from build123d import *

# Parameters (mm, degrees)
SKETCH1_W                = 154.8
SKETCH1_H                = 121.9997
SKETCH1_R                = 2.2
BOSS_EXTRUDE1_DEPTH      = 10
SKETCH2_W                = 184.8
SKETCH2_H                = 151.9997
SKETCH2_W_2              = 154.8
SKETCH2_H_2              = 121.9997
BOSS_EXTRUDE2_DEPTH      = 18
SKETCH2_2_W              = 184.8
SKETCH2_2_H              = 151.9997
SKETCH2_2_W_2            = 154.8
SKETCH2_2_H_2            = 121.9997
BOSS_EXTRUDE3_DEPTH      = 5
CUT_EXTRUDE1_DEPTH       = 229.604349915
CUT_EXTRUDE2_REACH       = 232.747
M5_CLEARANCE_HOLE1_D     = 5.5
M5_CLEARANCE_HOLE1_DEPTH = 23
M5_CLEARANCE_HOLE1_TIP   = 1.652366702
CUT_EXTRUDE3_DEPTH       = 6
CHAMFER1_SIZE            = 1
CHAMFER2_SIZE            = 3


with BuildPart() as part:
    # Sketch1 → Boss-Extrude1 (new body)
    with BuildSketch(Plane(origin=(0, 0, 0), x_dir=(1, 0, 0), z_dir=(0, 1, 0))):
        with Locations((77.4, 60.99985)):
            Rectangle(SKETCH1_W, SKETCH1_H)
        with Locations(Location((10, 53.3997, 0), (0, 0, 270))):
            Circle(SKETCH1_R, mode=Mode.SUBTRACT)
        with Locations(Location((10, 94.3997, 0), (0, 0, 270))):
            Circle(SKETCH1_R, mode=Mode.SUBTRACT)
        with Locations(Location((102, 94.3997, 0), (0, 0, 270))):
            Circle(SKETCH1_R, mode=Mode.SUBTRACT)
        with Locations(Location((102, 53.3997, 0), (0, 0, 270))):
            Circle(SKETCH1_R, mode=Mode.SUBTRACT)
        with BuildLine():
            Line((8, 49.3997), (8, 25.4))
            Line((8, 25.4), (104, 25.4))
            Line((104, 25.4), (104, 49.706462937))
            ThreePointArc((104, 49.706462937), (97.8, 53.3997), (104, 57.092937063))
            Line((104, 57.092937063), (104, 90.706462937))
            ThreePointArc((104, 90.706462937), (98.94961445, 91.512634363), (98.422291236, 96.5997))
            Line((98.422291236, 96.5997), (47, 96.5997))
            Line((47, 96.5997), (47, 49.3997))
            Line((47, 49.3997), (8, 49.3997))
        make_face(mode=Mode.SUBTRACT)
    extrude(amount=BOSS_EXTRUDE1_DEPTH)

    # Sketch2 → Boss-Extrude2 (add)
    with BuildSketch(Plane.XZ):
        with Locations((77.4, -60.99985)):
            Rectangle(SKETCH2_W, SKETCH2_H)
        with Locations((77.4, -60.99985)):
            Rectangle(SKETCH2_W_2, SKETCH2_H_2, mode=Mode.SUBTRACT)
    extrude(amount=-BOSS_EXTRUDE2_DEPTH)

    # Sketch2<2> → Boss-Extrude3 (add)
    # profile 1 of 2: a face of its own
    with BuildSketch(Plane.XZ):
        with Locations((77.4, -60.99985)):
            Rectangle(SKETCH2_2_W, SKETCH2_2_H)
        with Locations((77.4, -60.99985)):
            Rectangle(SKETCH2_2_W_2, SKETCH2_2_H_2, mode=Mode.SUBTRACT)
    # profile 2 of 2: a face of its own
    with BuildSketch(Plane.XZ):
        with Locations((77.4, -60.99985)):
            Rectangle(SKETCH2_2_W_2, SKETCH2_2_H_2)
    extrude(amount=BOSS_EXTRUDE3_DEPTH)

    # Sketch3 → Cut-Extrude1 (cut, through all)
    with BuildSketch(Plane.XY.offset(15)):
        with BuildLine():
            Line((52.4, 22), (102.4, 22))
            ThreePointArc((102.4, 22), (106.4, 18), (102.4, 14))
            Line((102.4, 14), (52.4, 14))
            ThreePointArc((52.4, 14), (48.4, 18), (52.4, 22))
        make_face()
    extrude(amount=-CUT_EXTRUDE1_DEPTH, mode=Mode.SUBTRACT)

    # Sketch4 → Cut-Extrude2 (cut, up to next)
    with BuildSketch(Plane(origin=(169.8, 0, 0), x_dir=(0, 0, -1), z_dir=(1, 0, 0)), mode=Mode.PRIVATE) as cut_extrude2_sk1:
        with BuildLine():
            Line((50.99985, 24), (70.99985, 24))
            ThreePointArc((70.99985, 24), (76.99985, 18), (70.99985, 12))
            Line((70.99985, 12), (50.99985, 12))
            ThreePointArc((50.99985, 12), (44.99985, 18), (50.99985, 24))
        make_face()
    cut_extrude2_tool1 = extrude(cut_extrude2_sk1.sketch, amount=-CUT_EXTRUDE2_REACH, mode=Mode.PRIVATE) & part.part
    add(cut_extrude2_tool1.solids().sort_by_distance((169.8, 18, -60.99985))[0], mode=Mode.SUBTRACT)

    # M5 Clearance Hole1
    with Locations(Plane(origin=(0, 18, 0), x_dir=(1, 0, 0), z_dir=(0, 1, 0))):
        with Locations((162.3, 129.4997), (162.3, -7.5), (-7.5, 129.4997), (-7.5, -7.5)):
            Hole(M5_CLEARANCE_HOLE1_D / 2, depth=M5_CLEARANCE_HOLE1_DEPTH)
            with Locations((0, 0, -(M5_CLEARANCE_HOLE1_DEPTH + M5_CLEARANCE_HOLE1_TIP / 2))):  # 118° drill point
                Cone(0, M5_CLEARANCE_HOLE1_D / 2, M5_CLEARANCE_HOLE1_TIP, mode=Mode.SUBTRACT)

    # Sketch7 → Cut-Extrude3 (cut)
    with BuildSketch(Plane.XZ.offset(5)):
        Polygon((-3.4, 9.867136104), (-7.5, 12.234272207), (-11.6, 9.867136104), (-11.6, 5.132863896), (-7.5, 2.765727793), (-3.4, 5.132863896), align=None)
        Polygon((158.2, 9.867136104), (158.2, 5.132863896), (162.3, 2.765727793), (166.4, 5.132863896), (166.4, 9.867136104), (162.3, 12.234272207), align=None)
        Polygon((158.2, -127.132563896), (158.2, -131.866836104), (162.3, -134.233972207), (166.4, -131.866836104), (166.4, -127.132563896), (162.3, -124.765427793), align=None)
        Polygon((-3.4, -127.132563896), (-7.5, -124.765427793), (-11.6, -127.132563896), (-11.6, -131.866836104), (-7.5, -134.233972207), (-3.4, -131.866836104), align=None)
    extrude(amount=-CUT_EXTRUDE3_DEPTH, mode=Mode.SUBTRACT)

    # Chamfer1
    chamfer1_edges = [part.edges().sort_by_distance(p)[0] for p in [
        (77.4, 14, 0),
        (77.4, 14, -121.9997),
        (49.571572875, 15.171572875, -121.9997),
        (49.571572875, 15.171572875, 0),
        (105.228427125, 15.171572875, 0),
        (105.228427125, 15.171572875, -121.9997),
        (154.8, 10, -60.99985),
        (154.8, 12, -60.99985),
        (154.8, 13.757359313, -46.757209313),
        (154.8, 13.757359313, -75.242490687),
        (77.4, 10, -121.9997),
        (27.5, 0, -49.3997),
        (47, 5, -49.3997),
        (8, 0, -37.39985),
        (8, 5, -49.3997),
        (56, 0, -25.4),
        (8, 5, -25.4),
        (104, 0, -37.553231469),
        (104, 5, -25.4),
        (97.8, 0, -53.3997),
        (104, 0, -73.8997),
        (98.94961445, 0, -91.512634363),
        (72.711145618, 0, -96.5997),
        (47, 0, -72.9997),
        (47, 5, -96.5997),
        (27.5, 10, -49.3997),
        (8, 10, -37.39985),
        (56, 10, -25.4),
        (104, 10, -37.553231469),
        (104, 10, -73.8997),
        (72.711145618, 10, -96.5997),
        (47, 10, -72.9997),
        (0, 10, -60.99985),
        (154.8, 14, 0),
        (0, 14, -121.9997),
        (0, 14, 0),
        (154.8, 14, -121.9997),
        (-15, 6.5, 15),
        (169.8, 6.5, 15),
        (169.8, 6.5, -136.9997),
        (-15, 6.5, -136.9997),
        (169.8, -5, -60.99985),
        (77.4, -5, 15),
        (77.4, 10, 0),
        (-15, -5, -60.99985),
        (77.4, -5, -136.9997),
    ]]
    chamfer(chamfer1_edges, length=CHAMFER1_SIZE - 0.0001)  # a hair under: the kernel refuses the full size

    # Chamfer2
    chamfer2_edges = [part.edges().sort_by_distance(p)[0] for p in [
        (77.4, 14, -136.9997),
        (49.571572875, 15.171572875, -136.9997),
        (105.228427125, 15.171572875, -136.9997),
        (49.571572875, 15.171572875, 15),
        (77.4, 14, 15),
        (105.228427125, 15.171572875, 15),
        (169.8, 13.757359313, -75.242490687),
        (169.8, 13.757359313, -46.757209313),
        (169.8, 12, -60.99985),
    ]]
    chamfer(chamfer2_edges, length=CHAMFER2_SIZE)


solid = part.part
Geometry check sheet. Reference: the model listing, model coordinates, mm. A direction names the side the tool comes from. Give positions to 0.01 mm unless a question says otherwise; leave off trailing zeros. Loops run counter-clockwise (first coordinate to the right, second up) from the corner with the lowest first, then second, coordinate; pieces in that order, holes last.
(1) Section check C-C on x = 57.5. Record the cut outline in (y, z), then the cut area to 3 significant figures.
From the geometry:
outline: (-5, -136) - (-4, -137) - (11, -137) - (14, -134) - (14, -123) - (13, -122) - (11, -122) - (10, -121) - (10, -97.6) - (9, -96.6) - (1, -96.6) - (0, -95.6) - (0, -26.4) - (1, -25.4) - (9, -25.4) - (10, -24.4) - (10, -1) - (11, 0) - (13, 0) - (14, 1) - (14, 12) - (11, 15) - (-4, 15) - (-5, 14) - close
area: 1,680 mm2
(2) Set-up check for faces 1 (the flat face through (-5.48, -2.04, 3.93)), 2 (the flat face through (10, 0, -94)), 3 (the conical face through (106.11, 14.37, -135.19)), 4 (the cylindrical face through (49.603, 15.141, 6.577)): record each of +Z, -Z, +X, -X, +Y, -Y from which the full face is reachable in a straight line by a thin tool's end or side.
From the geometry:
face 1: -Y
face 2: +Y
face 3: -Z, +Y
face 4: +Z, -Z, +Y
(3) Section check D-D on z = -103.5. Record the cut outline in (x, y).
From the geometry:
outline: (-15, -4) - (-14, -5) - (168.8, -5) - (169.8, -4) - (169.8, 18) - (154.8, 18) - (154.8, 11) - (153.8, 10) - (1, 10) - (0, 11) - (0, 18) - (-15, 18) - close
(4) Depth check by flat-ended pin: pin 1 Ø1.5 at (x, z) = (151, -18) entering from +Y; pin 2 Ø5.5 at (x, y) = (77.5, 14.5) entering from -Z; pin 3 Ø1.3 at (x, z) = (102, -94.5) entering from +Y. Enter the tip coordinate at first touch or a pass-through.
From the geometry:
pin 1: stops at y = 10
pin 2: stops at z = -136.25
pin 3: stops at y = 0
(5) Section check A-A on z = 7.5. Record the cut outline in (x, y).
From the geometry:
outline: (-15, -4) - (-14, -5) - (-11.6, -5) - (-11.6, 1) - (-10.25, 1) - (-10.25, 18) - (-15, 18) - close; (-4.75, 1) - (-3.4, 1) - (-3.4, -5) - (158.2, -5) - (158.2, 1) - (159.55, 1) - (159.55, 18) - (106.4, 18) arc R4 cw to (102.4, 14) - (52.4, 14) arc R4 cw to (48.4, 18) - (-4.75, 18) - close; (165.05, 1) - (166.4, 1) - (166.4, -5) - (168.8, -5) - (169.8, -4) - (169.8, 18) - (165.05, 18) - close
(6) Release check for a two-part mould opening along X. For faces 5 (the conical face through (167.95, 12.89, -46)), 6 (the flat face through (-15, 7, -62)), 7 (the flat face through (10, 0, -53)) record: released by +X, released by -X, zero draft, split by the parting line, or undercut.
From the geometry:
face 5: released by +X
face 6: released by -X
face 7: undercut
(7) Thickness scan on L1, parallel to Z at x = -7.5, y = 6.5; L2, parallel to Z at x = 14, y = 3.5; L3, parallel to Z at x = 96.5, y = 7.25. Record the ranges inside material, lowest first.
From the geometry:
L1: z = -137 to -132.25, -126.75 to 4.75, 10.25 to 15
L2: z = -137 to -49.4, -25.4 to 15
L3: z = -137 to -96.6, -25.4 to 15
